from build123d import *

# Parameters (mm, degrees)
SKETCH1_W                   = 63.5
SKETCH1_H                   = 749.3
BASE_FLANGE1_DEPTH          = 1.984375
F_1_2_0_5_DIAMETER_HOLE1_D  = 12.7
F_1_2_0_5_DIAMETER_HOLE2_D  = 12.7
EDGE_FLANGE2_DEPTH          = 749.3
EDGE_FLANGE2_BEND_DEPTH     = 749.3
F_10_0_201_DIAMETER_HOLE1_D = 4.9149
FILLET1_R                   = 12.7


# Sheet-metal steps are written as plain solids
with BuildPart() as part:
    # Sketch1 → Base-Flange1 (new body)
    with BuildSketch(Plane.XY):
        with Locations((0, 374.65)):
            Rectangle(SKETCH1_W, SKETCH1_H)
    extrude(amount=-BASE_FLANGE1_DEPTH)

    # 1/2 (0.5) Diameter Hole1 (through all)
    with Locations(Plane.XY):
        with Locations((-14.684375, 406.4), (14.684375, 406.4), (14.684375, 342.9), (-14.684375, 342.9)):
            Hole(F_1_2_0_5_DIAMETER_HOLE1_D / 2)

    # 1/2 (0.5) Diameter Hole2 (through all)
    with Locations(Plane.XY):
        with Locations((14.684375, 685.8), (14.684375, 736.6), (-14.684375, 736.6), (-14.684375, 685.8)):
            Hole(F_1_2_0_5_DIAMETER_HOLE2_D / 2)

    # Edge-Flange2 section (across the edge) → Edge-Flange2 (add)
    with BuildSketch(Plane(origin=(-33.734375, 749.3, 0), x_dir=(1, 0, 0), z_dir=(0, -1, 0))):
        with BuildLine():
            Line((-1.984375, 1.984375), (-1.984375, 19.05))
            Line((-1.984375, 19.05), (0, 19.05))
            Line((0, 19.05), (0, 1.984375))
            ThreePointArc((0, 1.984375), (0.581209981, 0.581209981), (1.984375, 0))
            Line((1.984375, 0), (1.984375, -1.984375))
            ThreePointArc((1.984375, -1.984375), (-0.821955038, -0.821955038), (-1.984375, 1.984375))
        make_face()
    extrude(amount=EDGE_FLANGE2_DEPTH)

    # Edge-Flange2 section 2 (across the edge) → Edge-Flange2 bend (add)
    with BuildSketch(Plane(origin=(33.734375, 0, 0), x_dir=(-1, 0, 0), z_dir=(0, 1, 0))):
        with BuildLine():
            Line((-1.984375, 1.984375), (-1.984375, 19.05))
            Line((-1.984375, 19.05), (0, 19.05))
            Line((0, 19.05), (0, 1.984375))
            ThreePointArc((0, 1.984375), (0.581209981, 0.581209981), (1.984375, 0))
            Line((1.984375, 0), (1.984375, -1.984375))
            ThreePointArc((1.984375, -1.984375), (-0.821955038, -0.821955038), (-1.984375, 1.984375))
        make_face()
    extrude(amount=EDGE_FLANGE2_BEND_DEPTH)

    # #10 (0.201) Diameter Hole1 (through all)
    with Locations(Plane(origin=(0, 0, -1.984375), x_dir=(-1, 0, 0), z_dir=(0, 0, -1))):
        with Locations((-14.684375, 19.05), (14.684375, 19.05), (-14.684375, 158.75), (14.684375, 158.75), (-14.684375, 311.15), (14.684375, 311.15), (-14.684375, 450.85), (14.684375, 450.85), (-14.684375, 660.4), (14.684375, 660.4)):
            Hole(F_10_0_201_DIAMETER_HOLE1_D / 2)

    # Fillet1
    fillet1_edges = [part.edges().sort_by_distance(p)[0] for p in [
        (-34.7265625, 749.3, 19.05),
        (-34.7265625, 0, 19.05),
        (34.7265625, 0, 19.05),
        (34.7265625, 749.3, 19.05),
    ]]
    fillet(fillet1_edges, radius=FILLET1_R)


solid = part.part
The listing builds one solid part. Answer for the finished solid, in the listing's coordinates (mm). A direction names the side the tool comes from. Give positions to 0.01 mm unless a question says otherwise; leave off trailing zeros. Order: outer loops, then holes, each group sorted by start corner. A loop starts at its lowest first (then second) coordinate and runs counter-clockwise, first axis right, second up. Notation, with made-up numbers: (45, -3.75) -> (97, -3.75) arc R17 ccw to (97, 27.25) -> close; hole circle Ø9 at (-9.75, 23). An arc over 180 degrees is marked (long way). Put each result on its own line as item: value.
Item 1: A cutting plane is placed at B-B on z = 12. Give the vertices of the cut face in (x, y).
Established:
outline: (-35.72, 1.33) -> (-33.73, 1.33) -> (-33.73, 747.97) -> (-35.72, 747.97) -> close; (33.73, 1.33) -> (35.72, 1.33) -> (35.72, 747.97) -> (33.73, 747.97) -> close
Item 2: Given P1, Ø6, axis at x = 27.5, y = 163.5, coming from the +Z side; P2, Ø10, axis at x = -14.68, y = 406.4, coming from the +Z side, each flat-ended and moving along its own axis, determine where each tip first touches the part or whether it passes through.
Established:
P1: stops at z = 0
P2: passes through
Item 3: A cutting plane is placed at C-C on y = 321. Give the vertices of the cut face in (x, z), plus the area to 3 significant figures.
Established:
outline: (-35.72, 1.98) arc R3.97 ccw to (-31.75, -1.98) -> (31.75, -1.98) arc R3.97 ccw to (35.72, 1.98) -> (35.72, 19.05) -> (33.73, 19.05) -> (33.73, 1.98) arc R1.98 cw to (31.75, 0) -> (-31.75, 0) arc R1.98 cw to (-33.73, 1.98) -> (-33.73, 19.05) -> (-35.72, 19.05) -> close
area: 212 mm^2
Item 4: For faces 4 (the face through (-33.734, 380, 11)), 5 (the face through (-13.9, 412.7, -1)), determine the directions among +Z, -Z, +X, -X, +Y, -Y from which every point of the face is accessible in a straight line to the end or side of a thin tool.
Established:
face 4: +Z, +Y, -Y
face 5: +Z, -Z
Item 5: Straight lines are drawn through the part: line 1 (X direction, y = 166.5, z = 7.75); line 2 (X direction, y = 158.75, z = -0.8); line 3 (X direction, y = 685.8, z = -0.95). For each, find the intervals that lie inside material, in ascending order.
Established:
line 1: x = -35.72 to -33.73, 33.73 to 35.72
line 2: x = -34.58 to -17.14, -12.23 to 12.23, 17.14 to 34.58
line 3: x = -34.42 to -21.03, -8.33 to 8.33, 21.03 to 34.42
Item 6: For a pull along Y with two mould halves and no side action, classify faces 1 (the face through (34.71, 3.82, 15.43)), 2 (the face through (16.06, 730.4, -1.01)), 3 (the face through (0, 380, 0)) as released by +Y, released by -Y, zero draft, split by the parting line, or undercut.
Established:
face 1: released by -Y
face 2: undercut
face 3: zero draft
Item 7: A cutting plane is placed at A-A on y = 406.4. Give the vertices of the cut face in (x, z).
Established:
outline: (-35.72, 1.98) arc R3.97 ccw to (-31.75, -1.98) -> (-21.03, -1.98) -> (-21.03, 0) -> (-31.75, 0) arc R1.98 cw to (-33.73, 1.98) -> (-33.73, 19.05) -> (-35.72, 19.05) -> close; (-8.33, -1.98) -> (8.33, -1.98) -> (8.33, 0) -> (-8.33, 0) -> close; (21.03, -1.98) -> (31.75, -1.98) arc R3.97 ccw to (35.72, 1.98) -> (35.72, 19.05) -> (33.73, 19.05) -> (33.73, 1.98) arc R1.98 cw to (31.75, 0) -> (21.03, 0) -> close
